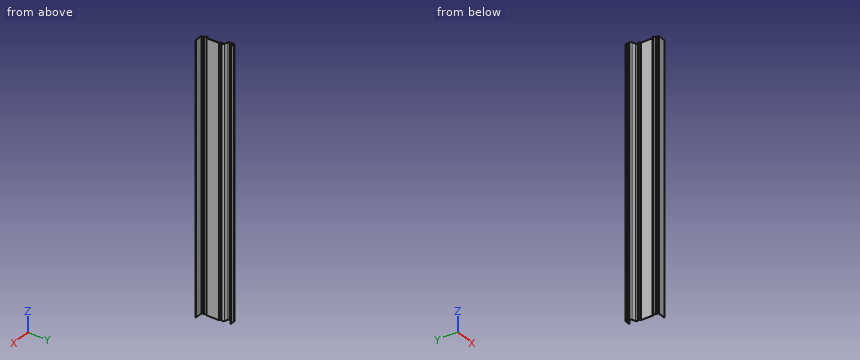
from build123d import *

# Parameters (mm, degrees)
EXTRUDE_THIN1_DEPTH = 1524
FILLET1_R           = 1.651


with BuildPart() as part:
    # Sketch1 → Extrude-Thin1 (new body)
    with BuildSketch(Plane.XY):
        with BuildLine():
            Line((0, 0), (-44.45, 0))
            Line((-44.45, 0), (-44.45, 12.7))
            Line((-44.45, 12.7), (-47.625, 12.7))
            Line((-47.625, 12.7), (-47.625, 16.725738686))
            ThreePointArc((-47.625, 16.725738686), (-49.543830542, 20.925868892), (-53.975, 22.225))
            Line((-53.975, 22.225), (-55.5625, 28.575))
            Line((-55.5625, 28.575), (-44.45, 31.75))
            Line((-44.45, 31.75), (-44.45, 101.6))
            ThreePointArc((-44.45, 101.6), (-47.130906672, 103.132600901), (-49.268021434, 105.361696367))
            ThreePointArc((-49.268021434, 105.361696367), (-51.342554678, 107.440960699), (-53.975, 108.74375))
            Line((-53.975, 108.74375), (-53.975, 113.50625))
            ThreePointArc((-53.975, 113.50625), (-47.702285259, 118.868550766), (-52.023643923, 125.898990228))
            Line((-52.023643923, 125.898990228), (-71.251525587, 132.108167244))
            ThreePointArc((-71.251525587, 132.108167244), (-76.113054084, 140.017411638), (-69.05625, 146.05))
            Line((-69.05625, 146.05), (-69.05625, 149.225))
            Line((-69.05625, 149.225), (-76.2, 149.225))
            Line((-76.2, 149.225), (-76.2, 165.1))
            Line((-76.2, 165.1), (-47.625, 165.1))
            Line((-47.625, 165.1), (-47.625, 163.449))
            Line((-47.625, 163.449), (-74.549, 163.449))
            Line((-74.549, 163.449), (-74.549, 150.876))
            Line((-74.549, 150.876), (-67.40525, 150.876))
            Line((-67.40525, 150.876), (-67.40525, 144.145))
            ThreePointArc((-67.40525, 144.145), (-74.289142714, 140.575721893), (-70.744173007, 133.679279703))
            Line((-70.744173007, 133.679279703), (-51.516291343, 127.470102687))
            ThreePointArc((-51.516291343, 127.470102687), (-45.984921685, 119.438339092), (-52.324, 112.027444216))
            Line((-52.324, 112.027444216), (-52.324, 109.890107647))
            ThreePointArc((-52.324, 109.890107647), (-49.883528392, 108.403175809), (-47.925046246, 106.322018525))
            ThreePointArc((-47.925046246, 106.322018525), (-45.671413632, 104.108692809), (-42.799, 102.794573098))
            Line((-42.799, 102.794573098), (-42.799, 30.504648368))
            Line((-42.799, 30.504648368), (-53.573493562, 27.426221636))
            Line((-53.573493562, 27.426221636), (-52.696098481, 23.916641311))
            ThreePointArc((-52.696098481, 23.916641311), (-47.916220995, 21.647519069), (-45.974, 16.725738686))
            Line((-45.974, 16.725738686), (-45.974, 14.351))
            Line((-45.974, 14.351), (-42.799, 14.351))
            Line((-42.799, 14.351), (-42.799, 1.651))
            Line((-42.799, 1.651), (0, 1.651))
            Line((0, 1.651), (0, 0))
        make_face()
    extrude(amount=-EXTRUDE_THIN1_DEPTH)

    # Fillet1
    fillet1_edges = [part.edges().sort_by_distance(p)[0] for p in [
        (-67.40525, 150.876, -762),
        (-67.40525, 144.145, -762),
        (-42.799, 102.794573098, -762),
        (-42.799, 30.504648368, -762),
        (-42.799, 14.351, -762),
        (-44.45, 0, -762),
        (-47.625, 12.7, -762),
        (-53.975, 22.225, -762),
        (-55.5625, 28.575, -762),
        (-53.975, 108.74375, -762),
        (-53.975, 113.50625, -762),
        (-76.2, 149.225, -762),
        (-76.2, 165.1, -762),
    ]]
    fillet(fillet1_edges, radius=FILLET1_R)


solid = part.part
Input: part model. Units: mm. Frame: model coordinates. Round coordinates to 2 decimals unless told otherwise and drop trailing zeros. Order: outer loops, then holes, each group sorted by start corner. A loop starts at its lowest first (then second) coordinate and runs counter-clockwise, first axis right, second up. Notation, with made-up numbers: (86, -2) - (140, -2) arc R24 cw to (140, 26) - close; hole circle Ø7 at (75.5, 50.25). An arc over 180 degrees is marked (long way). Use a Markdown table: item, result.
1. Section B-B on x = -18. Return the cut outline in (y, z).
Evaluation:
| item | result |
|---|---|
| outline | (0, -1524) - (1.65, -1524) - (1.65, 0) - (0, 0) - close |
2. Section A-A on y = 50.5. Return the cut outline in (x, z), then the cut area to 3 significant figures.
Evaluation:
| item | result |
|---|---|
| outline | (-44.45, -1524) - (-42.8, -1524) - (-42.8, 0) - (-44.45, 0) - close |
| area | 2,520 mm^2 |
3. Material intervals for probe 1 along Y at (x, z) = (-71.5, -69) (3 decimals); probe 2 along Y at (x, z) = (-5, -457); probe 3 along Y at (x, z) = (-56, -377), sorted ascending.
Evaluation:
| item | result |
|---|---|
| probe 1 | 132.193 to 133.987, 143.825 to 145.619, 149.225 to 150.876, 163.449 to 165.1 |
| probe 2 | 0 to 1.65 |
| probe 3 | 127.18 to 128.92, 163.45 to 165.1 |
4. First-contact query: pin 1 (6 mm diameter, centred on y = 23.5, z = -707, fed in from -X); pin 2 (1.1 mm diameter, centred on y = 110.5, z = -510.5, fed in from +X); pin 3 (1.9 mm diameter, centred on y = 15.5, z = -673, fed in from +X). Flat tips, straight axial feed; report the tip coordinate or a pass-through.
Evaluation:
| item | result |
|---|---|
| pin 1 | x = -55.04 |
| pin 2 | x = -52.32 |
| pin 3 | x = -45.97 |
